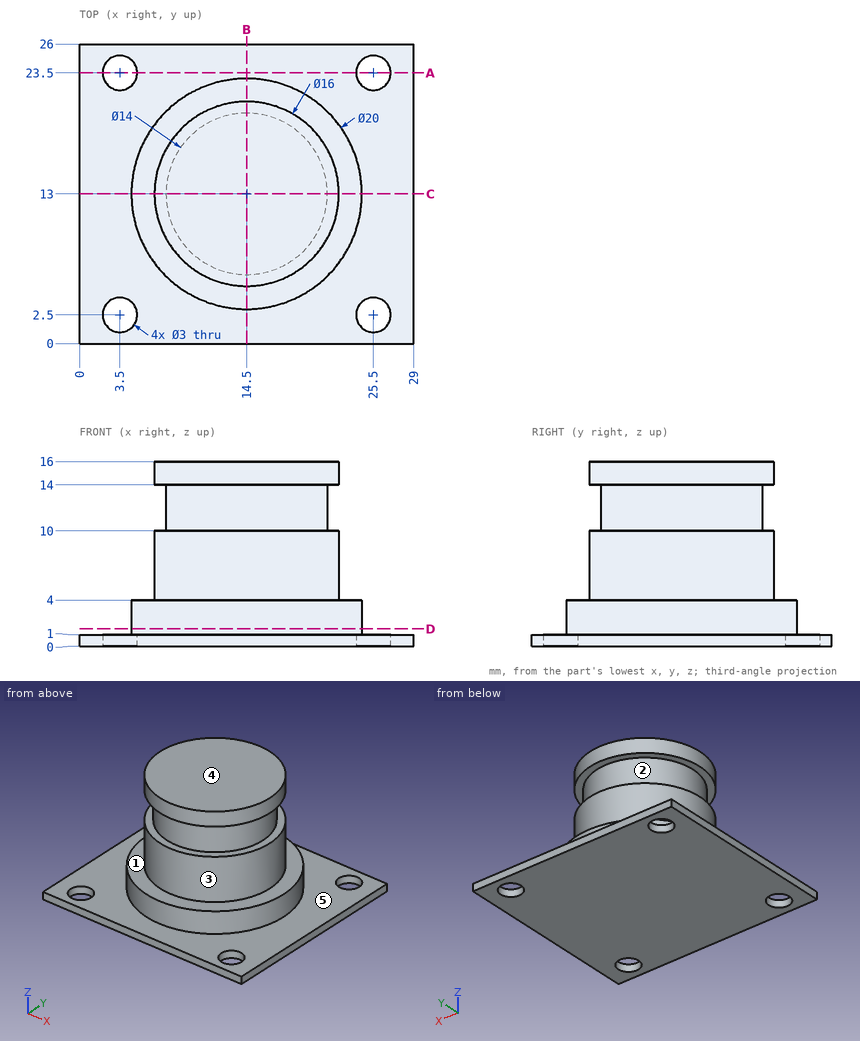
Source: three-view drawing plus pictorial views. Frame: mm from the lowest corner of the part. A direction names the side the tool comes from. Round coordinates to 2 decimals unless told otherwise and drop trailing zeros. Order: outer loops, then holes, each group sorted by start corner. A loop starts at its lowest first (then second) coordinate and runs counter-clockwise, first axis right, second up. Notation, with made-up numbers: (82, 31.5) -> (115, 31.5) arc R20 ccw to (115, 35.5) -> close; hole circle Ø10 at (-5.5, -33.5). An arc over 180 degrees is marked (long way). Use one line per item in the form item = value.
(1) Section C-C on y = 13. Return loops of the section in (x, z), and give its area (3 significant figures).
Results list:
outline = (0, 0) -> (29, 0) -> (29, 1) -> (24.5, 1) -> (24.5, 4) -> (22.5, 4) -> (22.5, 10) -> (21.5, 10) -> (21.5, 14) -> (22.5, 14) -> (22.5, 16) -> (6.5, 16) -> (6.5, 14) -> (7.5, 14) -> (7.5, 10) -> (6.5, 10) -> (6.5, 4) -> (4.5, 4) -> (4.5, 1) -> (0, 1) -> close
area = 273 mm^2
(2) Draft query along Z for the marked faces 1, 2 and 3. Return one class per face: pulls with the +Z half, pulls with the -Z half, needs draft (parallel to the pull), parting line crosses it, or undercut.
Results list:
face_1 = pulls with the +Z half
face_2 = undercut
face_3 = needs draft
(3) Section D-D on z = 1.5. Return loops of the section in (x, y).
Results list:
outline = circle Ø20 at (14.5, 13)
(4) Ray query, probe 1 along Y at (x, z) = (25.5, 0.3); probe 2 along Z at (x, y) = (22.75, 21); probe 3 along Z at (x, y) = (14, 22.25). Return the intervals inside material, ascending. Write a range as [from, to].
Results list:
probe_1 = [0, 1], [4, 22], [25, 26]
probe_2 = [0, 1]
probe_3 = [0, 4]
(5) Section A-A on y = 23.5. Return loops of the section in (x, z), and give its area (3 significant figures).
Results list:
outline = (0, 0) -> (2, 0) -> (2, 1) -> (0, 1) -> close; (5, 0) -> (24, 0) -> (24, 1) -> (5, 1) -> close; (27, 0) -> (29, 0) -> (29, 1) -> (27, 1) -> close
area = 23.0 mm^2
(6) First-contact query: pin 1 Ø5 at (x, z) = (17.5, 8) entering from -Y; pin 2 Ø3 at (x, z) = (7, 13) entering from -Y; pin 3 Ø4 at (x, z) = (21.5, 8.5) entering from -Y (3 decimals); pin 4 Ø1.8 at (x, y) = (25.5, 23.5) entering from +Z. Flat tips, straight axial feed; report the tip coordinate or a pass-through.
Results list:
pin_1 = 5.02
pin_2 = 8.18
pin_3 = 6.755
pin_4 = through
(7) Access query for the marked faces 4 and 5. Directions: +Z, -Z, +X, -X, +Y, -Y. A direction counts if a zero-diameter tool reaches every point of the face in a straight line with its end or side. Return the directions, or none.
Results list:
face_4 = +Z, +X, -X, +Y, -Y
face_5 = +Z
(8) Section B-B on x = 14.5. Return loops of the section in (y, z), and give its area (3 significant figures).
Results list:
outline = (0, 0) -> (26, 0) -> (26, 1) -> (23, 1) -> (23, 4) -> (21, 4) -> (21, 10) -> (20, 10) -> (20, 14) -> (21, 14) -> (21, 16) -> (5, 16) -> (5, 14) -> (6, 14) -> (6, 10) -> (5, 10) -> (5, 4) -> (3, 4) -> (3, 1) -> (0, 1) -> close
area = 270 mm^2
